Input: part model. Units: mm. Frame: model coordinates. A direction names the side the tool comes from. Round coordinates to 2 decimals unless told otherwise and drop trailing zeros. Put each result on its own line as item: value. Start each with the question number.
1) Section A-A on y = 195. State how many separate pieces and enclosed holes the cut face has, plus the area to 3 significant figures.
2) Pin query (flat end, axial travel): pin 1 (2 mm diameter, centred on x = 14.5, y = 125, fed in from +Z); pin 2 (1.7 mm diameter, centred on y = 146.5, z = -16, fed in from -X); pin 3 (0.6 mm diameter, centred on y = 165.5, z = -29, fed in from +X). Return the tip coordinate at first contact, or that it passes through.
3) Reachability of faces 5 (the face through (15, 123, -19)), 6 (the face through (30, 123, -23)), 7 (the face through (28, 123, -9)) from +Z, -Z, +X, -X, +Y, -Y: full face, straight path, thin tool, end or side. Return the list, or none.
4) Line query: probe 1 along Z at (x, y) = (4.75, 89); probe 2 along X at (y, z) = (55, -3.5); probe 3 along Z at (x, y) = (11.5, 208.5). Output: solid intervals per line, ascending.
5) Draft query along X for faces 1 (the face through (19, 123, -15)), 2 (the face through (0, 123, -7)), 3 (the face through (26, 123, -7)), 4 (the face through (9, 123, -2)). Return one class per face: +X half, -X half, draft (parallel to the pull), parting line (faces both ways), or undercut.
from build123d import *

# Parameters (mm, degrees)
BOSS_EXTRUDE1_DEPTH = 250


with BuildPart() as part:
    # Sketch1 → Boss-Extrude1 (new body)
    with BuildSketch(Plane(origin=(0, 0, 0), x_dir=(1, 0, 0), z_dir=(0, 1, 0))):
        with BuildLine():
            Line((0, 28), (0, 18.4))
            Line((0, 18.4), (2, 18.4))
            Line((2, 18.4), (2, 23))
            Line((2, 23), (5.833273811, 23))
            Line((5.833273811, 23), (11, 17.833273811))
            Line((11, 17.833273811), (11, 15))
            Line((11, 15), (11, 12.166726189))
            Line((11, 12.166726189), (5.833273811, 7))
            Line((5.833273811, 7), (2, 7))
            Line((2, 7), (2, 11.6))
            Line((2, 11.6), (0, 11.6))
            Line((0, 11.6), (0, 2))
            ThreePointArc((0, 2), (0.585786438, 0.585786438), (2, 0))
            Line((2, 0), (11.6, 0))
            Line((11.6, 0), (11.6, 2))
            Line((11.6, 2), (7, 2))
            Line((7, 2), (7, 5.833273811))
            Line((7, 5.833273811), (12.166726189, 11))
            Line((12.166726189, 11), (15, 11))
            Line((15, 11), (17.833273811, 11))
            Line((17.833273811, 11), (23, 5.833273811))
            Line((23, 5.833273811), (23, 2))
            Line((23, 2), (18.4, 2))
            Line((18.4, 2), (18.4, 0))
            Line((18.4, 0), (28, 0))
            ThreePointArc((28, 0), (29.414213562, 0.585786438), (30, 2))
            Line((30, 2), (30, 11.6))
            Line((30, 11.6), (28, 11.6))
            Line((28, 11.6), (28, 7))
            Line((28, 7), (24.166726189, 7))
            Line((24.166726189, 7), (19, 12.166726189))
            Line((19, 12.166726189), (19, 15))
            Line((19, 15), (19, 17.833273811))
            Line((19, 17.833273811), (24.166726189, 23))
            Line((24.166726189, 23), (28, 23))
            Line((28, 23), (28, 18.4))
            Line((28, 18.4), (30, 18.4))
            Line((30, 18.4), (30, 28))
            ThreePointArc((30, 28), (29.414213562, 29.414213562), (28, 30))
            Line((28, 30), (18.4, 30))
            Line((18.4, 30), (18.4, 28))
            Line((18.4, 28), (23, 28))
            Line((23, 28), (23, 24.166726189))
            Line((23, 24.166726189), (17.833273811, 19))
            Line((17.833273811, 19), (15, 19))
            Line((15, 19), (12.166726189, 19))
            Line((12.166726189, 19), (7, 24.166726189))
            Line((7, 24.166726189), (7, 28))
            Line((7, 28), (11.6, 28))
            Line((11.6, 28), (11.6, 30))
            Line((11.6, 30), (2, 30))
            ThreePointArc((2, 30), (0.585786438, 29.414213562), (0, 28))
        make_face()
        with BuildLine():
            Line((6, 28.4), (6, 24))
            Line((6, 24), (1.6, 24))
            Line((1.6, 24), (1.6, 26.8))
            ThreePointArc((1.6, 26.8), (2.06862915, 27.93137085), (3.2, 28.4))
            Line((3.2, 28.4), (6, 28.4))
        make_face(mode=Mode.SUBTRACT)
        with BuildLine():
            Line((26.8, 28.4), (24, 28.4))
            Line((24, 28.4), (24, 24))
            Line((24, 24), (28.4, 24))
            Line((28.4, 24), (28.4, 26.8))
            ThreePointArc((28.4, 26.8), (27.93137085, 27.93137085), (26.8, 28.4))
        make_face(mode=Mode.SUBTRACT)
        with BuildLine():
            Line((28.4, 3.2), (28.4, 6))
            Line((28.4, 6), (24, 6))
            Line((24, 6), (24, 1.6))
            Line((24, 1.6), (26.8, 1.6))
            ThreePointArc((26.8, 1.6), (27.93137085, 2.06862915), (28.4, 3.2))
        make_face(mode=Mode.SUBTRACT)
        with BuildLine():
            Line((3.2, 1.6), (6, 1.6))
            Line((6, 1.6), (6, 6))
            Line((6, 6), (1.6, 6))
            Line((1.6, 6), (1.6, 3.2))
            ThreePointArc((1.6, 3.2), (2.06862915, 2.06862915), (3.2, 1.6))
        make_face(mode=Mode.SUBTRACT)
        with BuildLine():
            ThreePointArc((15, 17.5), (13.232233047, 16.767766953), (12.5, 15))
            ThreePointArc((12.5, 15), (13.232233047, 13.232233047), (15, 12.5))
            ThreePointArc((15, 12.5), (16.767766953, 13.232233047), (17.5, 15))
            ThreePointArc((17.5, 15), (16.767766953, 16.767766953), (15, 17.5))
        make_face(mode=Mode.SUBTRACT)
    extrude(amount=BOSS_EXTRUDE1_DEPTH)


solid = part.part
Geometry results:
1. separate pieces: 1
1. enclosed holes: 5
1. area: 278 mm²
2. pin 1: stops at z = -11
2. pin 2: stops at x = 11
2. pin 3: stops at x = 29.87
3. face 5: -Z, +Y, -Y
3. face 6: +Z, -Z, +X, +Y, -Y
3. face 7: +Y, -Y
4. probe 1: z = -30 to -28.4, -24 to -23, -7 to -6, -1.6 to 0
4. probe 2: x = 0 to 1.6, 6 to 7, 23 to 24, 28.4 to 30
4. probe 3: z = -30 to -28, -19.67 to -10.33, -2 to 0
5. face 1: +X half
5. face 2: -X half
5. face 3: undercut
5. face 4: undercut
